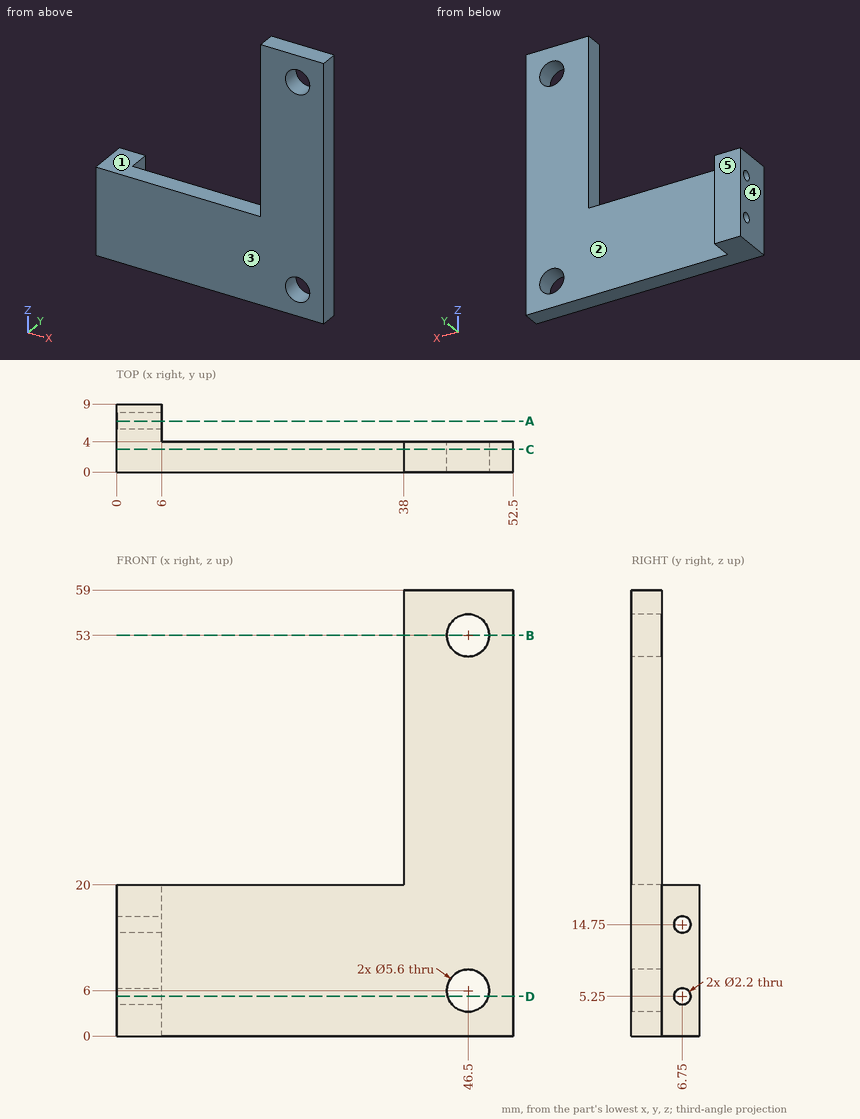
Part print with two shaded views. Sizes in mm from the minimum x, y, z corner. A direction names the side the tool comes from. Coordinates: 2 decimals unless noted, no trailing zeros. Order: outer loops, then holes, each group sorted by start corner. A loop starts at its lowest first (then second) coordinate and runs counter-clockwise, first axis right, second up. Notation, with made-up numbers: (-38.75, 48.5) - (-14.75, 48.5) arc R25 cw to (-14.75, 65.5) - close; hole circle Ø11 at (-29, 24.25). An arc over 180 degrees is marked (long way). Write item = value, one per line. Start each with the question number.
1) Two-plate mould, pull along X, no slides. Class the marked faces 4 and 5: pulls with the +X half, pulls with the -X half, needs draft (parallel to the pull), parting line crosses it, or undercut.
2) 3-axis set-ups, long thin cutter, end or side, ignore diameter. For the marked faces 1, 2 and 3: which of +Z, -Z, +X, -X, +Y, -Y reach the whole face in a straight line?
3) Flat gauge pins, fed straight in: pin 1 Ø5 at (y, z) = (2.5, 51) entering from -X; pin 2 Ø23 at (x, z) = (34, 41.5) entering from +Y; pin 3 Ø2.5 at (y, z) = (6, 8.5) entering from +X. Where does each tip first touch, or does it go through?
4) Wall check: line 1 along Z through (x, y) = (1.4, 6.75); line 2 along Z through (x, y) = (46.5, 2.5); line 3 along X through (y, z) = (3.25, 53). Give the ranges that are in metal, low to high. Write a range as from..to.
5) Saw through at A-A on y = 6.75. Write the cut outline in (x, z), then the cut area to 3 significant figures.
6) Saw through at C-C on y = 3. Write the cut outline in (x, z), then the cut area to 3 significant figures.
7) Saw through at D-D on z = 5.25. Write the cut outline in (x, y).
8) Saw through at B-B on z = 53. Write the cut outline in (x, y), then the cut area to 3 significant figures.
From the geometry:
q1.face_4 = pulls with the -X half
q1.face_5 = needs draft
q2.face_1 = +Z, -X, +Y, -Y
q2.face_2 = +Z, -Z, +X, +Y
q2.face_3 = +Z, -Z, +X, -X, -Y
q3.pin_1 = 38
q3.pin_2 = 4
q3.pin_3 = 6
q4.line_1 = 0..4.15, 6.35..13.65, 15.85..20
q4.line_2 = 0..3.2, 8.8..50.2, 55.8..59
q4.line_3 = 38..43.7, 49.3..52.5
q5.outline = (0, 0) - (6, 0) - (6, 4.15) - (0, 4.15) - close; (0, 6.35) - (6, 6.35) - (6, 13.65) - (0, 13.65) - close; (0, 15.85) - (6, 15.85) - (6, 20) - (0, 20) - close
q5.area = 93.6 mm^2
q6.outline = (0, 0) - (52.5, 0) - (52.5, 59) - (38, 59) - (38, 20) - (0, 20) - close; hole circle Ø5.6 at (46.5, 6); hole circle Ø5.6 at (46.5, 53)
q6.area = 1,570 mm^2
q7.outline = (0, 0) - (43.8, 0) - (43.8, 4) - (6, 4) - (6, 5.65) - (0, 5.65) - close; (0, 7.85) - (6, 7.85) - (6, 9) - (0, 9) - close; (49.2, 0) - (52.5, 0) - (52.5, 4) - (49.2, 4) - close
q8.outline = (38, 0) - (43.7, 0) - (43.7, 4) - (38, 4) - close; (49.3, 0) - (52.5, 0) - (52.5, 4) - (49.3, 4) - close
q8.area = 35.6 mm^2
